Read the model definition and answer for the solid it produces. Units are mm, in the model's axes. A direction names the side the tool comes from. Coordinates: 2 decimals unless noted, no trailing zeros. Write each loop counter-clockwise with the first axis right and the second up, starting at its lowest first coordinate (ties: lowest second). Pieces come first, ordered by that corner, then holes.
Item 1: Determine the mould class of faces 6 (the face through (13, 17, -177.8)), 7 (the face through (22.817, 20.876, -3.488)), 8 (the face through (13, 16.129, -166)) for opening direction Y: released by +Y, released by -Y, zero draft, split by the parting line, or undercut.
Item 2: A tool of negligible diameter and unlimited length cuts with its end or side. For faces 1 (the face through (23, 23, -6.096)), 2 (the face through (13, 17, 0)), 3 (the face through (3, 25.908, -3)), 4 (the face through (3.175, 8, -88)), 5 (the face through (6.096, 25, -2)), from which of +Z, -Z, +X, -X, +Y, -Y can it reach the whole face along a straight path? Write none if from no direction.
Item 3: Each of these flat-tipped pins is pushed along its axis until it touches: P1, Ø1.5, axis at y = 23, z = -156, coming from the +X side; P2, Ø3, axis at x = 10, z = -121, coming from the -Y side; P3, Ø6, axis at x = 2.5, y = 22, coming from the -Z side; P4, Ø3, axis at x = 21.5, y = 22.5, coming from the -Z side. Where does it stop, or does it pass through?
Item 4: Section C-C (y = 22.86) is taken. Give the vertices of the cut face in (x, z).
Item 5: Section D-D (z = -97) is taken. Give the vertices of the cut face in (x, y) (3 decimals), then the cut area to 3 significant figures.
Item 6: Section B-B (x = 13) is taken. Give the vertices of the cut face in (y, z), then the cut area to 3 significant figures.
Item 7: Section A-A (y = 5) is taken. Give the vertices of the cut face in (x, z) (3 decimals), then the cut area to 3 significant figures.
Item 8: Straight lines are drawn through the part: probe 1 along X at (y, z) = (7, -29.5) (3 decimals); probe 2 along Z at (x, y) = (3.5, 22.86); probe 3 along Z at (x, y) = (2.25, 13.75). For each, find the intervals that lie inside material, in ascending order.
from build123d import *

# Parameters (mm, degrees)
BOSS_EXTRUDE2_DEPTH     = 177.8
SKETCH19_R              = 2.032
CUT_EXTRUDE3_DEPTH      = 26.908
SKETCH21_W              = 6.096
SKETCH21_H              = 6.096
BOSS_EXTRUDE4_DEPTH     = 5.588
SKETCH22_R              = 2.032
CUT_EXTRUDE4_DEPTH      = 20.812
CUT_EXTRUDE4_DEPTH_BACK = 7.096


with BuildPart() as part:
    # Sketch2 → Boss-Extrude2 (new body)
    with BuildSketch(Plane.XY):
        Polygon((0, 0), (0, 20.32), (25.908, 20.32), (25.908, 0), (22.733, 0), (22.733, 16.129), (3.175, 16.129), (3.175, 0), align=None)
    extrude(amount=-BOSS_EXTRUDE2_DEPTH)

    # Sketch19 → Cut-Extrude3 (cut, through all)
    with BuildSketch(Plane(origin=(0, 0, 0), x_dir=(0, 0, -1), z_dir=(1, 0, 0))):
        with Locations((24.13, 14.224)):
            Circle(SKETCH19_R)
        with Locations((64.77, 14.224)):
            Circle(SKETCH19_R)
        with Locations((113.03, 14.224)):
            Circle(SKETCH19_R)
        with Locations((153.67, 14.224)):
            Circle(SKETCH19_R)
    extrude(amount=CUT_EXTRUDE3_DEPTH, mode=Mode.SUBTRACT)

    # Sketch21 → Boss-Extrude4 (add)
    with BuildSketch(Plane(origin=(0, 20.32, 0), x_dir=(1, 0, 0), z_dir=(0, 1, 0))):
        with Locations((3.048, 3.048)):
            Rectangle(SKETCH21_W, SKETCH21_H)
        with Locations((22.86, 3.048)):
            Rectangle(SKETCH21_W, SKETCH21_H)
    extrude(amount=BOSS_EXTRUDE4_DEPTH)

    # Sketch22 → Cut-Extrude4 (cut, two sides)
    with BuildSketch(Plane.ZY.offset(-19.812)) as cut_extrude4_sk:
        with Locations((-3.048, 22.86)):
            Circle(SKETCH22_R)
    extrude(amount=CUT_EXTRUDE4_DEPTH, mode=Mode.SUBTRACT)
    extrude(cut_extrude4_sk.sketch, amount=-CUT_EXTRUDE4_DEPTH_BACK, mode=Mode.SUBTRACT)


solid = part.part
Established:
1. face 6: zero draft
1. face 7: undercut
1. face 8: released by -Y
2. face 1: -Z, +X, -X, +Y
2. face 2: +Z, +X, -X, +Y, -Y
2. face 3: +Z, -Z, +X, -X, +Y
2. face 4: +Z, -Z, -Y
2. face 5: +Z, -Z, +Y
3. P1: passes through
3. P2: stops at y = 16.13
3. P3: stops at z = -177.8
3. P4: stops at z = -6.1
4. outline: (0, -6.1) - (6.1, -6.1) - (6.1, -5.08) - (0, -5.08) - close; (0, -1.02) - (6.1, -1.02) - (6.1, 0) - (0, 0) - close; (19.81, -6.1) - (25.91, -6.1) - (25.91, -5.08) - (19.81, -5.08) - close; (19.81, -1.02) - (25.91, -1.02) - (25.91, 0) - (19.81, 0) - close
5. outline: (0, 0) - (3.175, 0) - (3.175, 16.129) - (22.733, 16.129) - (22.733, 0) - (25.908, 0) - (25.908, 20.32) - (0, 20.32) - close
5. area: 211 mm2
6. outline: (16.13, -177.8) - (20.32, -177.8) - (20.32, 0) - (16.13, 0) - (16.13, -23.42) arc R2.03 cw to (16.13, -24.84) - (16.13, -64.06) arc R2.03 cw to (16.13, -65.48) - (16.13, -112.32) arc R2.03 cw to (16.13, -113.74) - (16.13, -152.96) arc R2.03 cw to (16.13, -154.38) - close
6. area: 745 mm2
7. outline: (0, -177.8) - (3.175, -177.8) - (3.175, 0) - (0, 0) - close; (22.733, -177.8) - (25.908, -177.8) - (25.908, 0) - (22.733, 0) - close
7. area: 1,130 mm2
8. probe 1: x = 0 to 3.175, 22.733 to 25.908
8. probe 2: z = -6.1 to -5.08, -1.02 to 0
8. probe 3: z = -177.8 to -155.65, -151.69 to -115.01, -111.05 to -66.75, -62.79 to -26.11, -22.15 to 0
